Autodesk Inventor part; units mm, degrees
ref_plane "YZ Plane" through (0, 0, 0) normal (1, 0, 0) x (0, 1, 0)
ref_plane "XZ Plane" through (0, 0, 0) normal (0, 1, 0) x (-1, 0, 0)
ref_plane "XY Plane" through (0, 0, 0) normal (0, 0, 1) x (1, 0, 0)
sketch "Sketch1" plane through (0, 0, 0) normal (0, 0, 1) x (1, 0, 0)
  line L0 (-35.56, 38.35) -> (-35.56, 5)
  line L1 (0, 5) -> (0, 38.35)
  line L2 (-37.78, 47.225) -> (2.22, 47.225)
  line L3 (2.22, -2.775) -> (-37.78, -2.775)
  line L4 (-37.78, -2.775) -> (-37.78, 47.225)
  line L5 (1.22, 24.725) -> (1.22, 19.725)
  line L6 (1.22, 19.725) -> (2.22, 19.725)
  line L7 (2.22, 24.725) -> (1.22, 24.725)
  line L8 (2.22, 47.225) -> (2.22, 24.725)
  line L9 (2.22, 19.725) -> (2.22, -2.775)
  circle A0 centre (-3.05, 41.4) radius 1.4
  circle A1 centre (-32.51, 41.4) radius 1.4
  arc A2 (-6.1, 41.4) -> (-3.05, 38.35) centre (-3.05, 41.4) ccw
  line L10 (-6.1, 41.4) -> (-6.1, 44.45)
  line L11 (-3.05, 38.35) -> (0, 38.35)
  arc A3 (-32.51, 38.35) -> (-29.46, 41.4) centre (-32.51, 41.4) ccw
  line L12 (-29.46, 41.4) -> (-29.46, 44.45)
  line L13 (-32.51, 38.35) -> (-35.56, 38.35)
  line L14 (-6.1, 44.45) -> (-29.46, 44.45)
  line L15 (-35.56, 5) -> (0, 5)
  line L16 (0, 38.35) -> (0, 44.45)
  line L17 (0, 44.45) -> (-6.1, 44.45)
  line L18 (-29.46, 44.45) -> (-35.56, 44.45)
  line L19 (-35.56, 44.45) -> (-35.56, 38.35)
  line L20 (0, 5) -> (-35.56, 5)
  line L21 (-35.56, 5) -> (-35.56, -0.1476)
  line L22 (-35.56, -0.1476) -> (0, -0.1476)
  line L23 (0, -0.1476) -> (0, 5)
  point P0 (-17.78, 22.225)
  dimension "d0" = 40
  dimension "d1" = 50
  dimension "d2" = 5
  dimension "d4" = 1
  dimension "d6" = 7.775
  dimension "d8" = 3.05
  dimension "d9" = 2.8
extrude "Extrusion1" add sketch "Sketch1" along normal blind 5 contours L2 L8 L7 L5 L6 L9 L3 L4
ref_plane "Work Plane1" through (0, 0, 0) normal (0, 0, 1) x (1, 0, 0)
sketch "Sketch2" plane through (0, 0, 0) normal (0, 0, 1) x (1, 0, 0)
  line L0 (-35.56, 38.35) -> (-35.56, 5)
  line L1 (0, 5) -> (0, 38.35)
  line L2 (-37.78, 47.225) -> (2.22, 47.225)
  line L3 (2.22, -2.775) -> (-37.78, -2.775)
  line L4 (-37.78, -2.775) -> (-37.78, 47.225)
  line L5 (1.22, 24.725) -> (1.22, 19.725)
  line L6 (1.22, 19.725) -> (2.22, 19.725)
  line L7 (2.22, 24.725) -> (1.22, 24.725)
  line L8 (2.22, 47.225) -> (2.22, 24.725)
  line L9 (2.22, 19.725) -> (2.22, -2.775)
  circle A0 centre (-3.05, 41.4) radius 1.4
  circle A1 centre (-32.51, 41.4) radius 1.4
  arc A2 (-6.1, 41.4) -> (-3.05, 38.35) centre (-3.05, 41.4) ccw
  line L10 (-6.1, 41.4) -> (-6.1, 44.45)
  line L11 (-3.05, 38.35) -> (0, 38.35)
  arc A3 (-32.51, 38.35) -> (-29.46, 41.4) centre (-32.51, 41.4) ccw
  line L12 (-29.46, 41.4) -> (-29.46, 44.45)
  line L13 (-32.51, 38.35) -> (-35.56, 38.35)
  line L14 (-6.1, 44.45) -> (-29.46, 44.45)
  line L15 (-35.56, 5) -> (0, 5)
  line L16 (0, 38.35) -> (0, 44.45)
  line L17 (0, 44.45) -> (-6.1, 44.45)
  line L18 (-29.46, 44.45) -> (-35.56, 44.45)
  line L19 (-35.56, 44.45) -> (-35.56, 38.35)
  line L20 (0, 5) -> (-35.56, 5)
  line L21 (-35.56, 5) -> (-35.56, -0.2)
  line L22 (-35.56, -0.2) -> (0, -0.2)
  line L23 (0, -0.2) -> (0, 5)
  line L24 (-35.56, -0.1476) -> (0, -0.1476)
  point P0 (0, 0)
  point P1 (-17.78, 22.225)
  dimension "d12" = 40
  dimension "d13" = 50
  dimension "d14" = 5
  dimension "d15" = 1
  dimension "d16" = 7.775
  dimension "d17" = 3.05
  dimension "d18" = 2.8
  dimension "d27" = 5.2
extrude "Extrusion2" add sketch "Sketch2" along normal blind 2 contours L19 L18 L12 A3 L13 | L15 L23 L24 L21 | L24 L23 L22 L21 | L11 A2 L10 L17 L16
sketch "Sketch3" plane through (-37.78, -2.775, 0) normal (-1, 0, 0) x (0, 0, 1)
  line L0 (5.9421, 36.5891) -> (1.9421, 36.5891)
  line L1 (1.9421, 36.5891) -> (1.9421, 23.5891)
  line L2 (1.9421, 23.5891) -> (5.9421, 23.5891)
  line L3 (5.9421, 23.5891) -> (5.9421, 36.5891)
  point P0 (0, 2.775)
  dimension "d21" = 4
  dimension "d22" = 13
extrude "Extrusion3" cut sketch "Sketch3" against normal up to surface (2.22 mm away)
sketch "Sketch4" plane through (0, 0, 0) normal (0, 0, -1) x (-1, 0, 0)
  line L0 (9.525, 39.121) -> (2.794, 39.121)
  line L1 (2.794, 39.121) -> (2.0566, 39.0072)
  line L2 (2.0566, 39.0072) -> (1.3738, 38.7064)
  arc A0 (29.46, 41.4) -> (32.51, 38.35) centre (32.51, 41.4) ccw
  line L3 (30.483, 39.121) -> (32.766, 39.121)
  line L4 (35.56, 38.35) -> (32.51, 38.35)
  arc A1 (34.63, 38.35) -> (32.766, 39.121) centre (32.5832, 36.0404) ccw
  line L5 (34.63, 38.35) -> (32.51, 38.35)
  arc A2 (30.483, 39.121) -> (32.51, 38.35) centre (32.51, 41.4) ccw
  arc A3 (3.05, 38.35) -> (6.1, 41.4) centre (3.05, 41.4) ccw
  arc A4 (3.05, 38.35) -> (5.1075, 39.121) centre (3.078, 41.4062) ccw
  arc A5 (2.794, 39.121) -> (0.93, 38.35) centre (2.917, 36.1849) ccw
  line L6 (5.1075, 39.121) -> (2.794, 39.121)
  line L7 (3.05, 38.35) -> (0.93, 38.35)
  point P0 (0, 0)
extrude "Extrusion4" cut sketch "Sketch4" against normal blind 2 contours A4 A3 L0 | A3 L7 A5 L2 L1 L0 | L1 A5 | A5 L2 | L3 A1 L4 A0
sketch "Sketch5" plane through (0, 0, 0) normal (0, 0, -1) x (-1, 0, 0)
  line L0 (26.712, -2.7097) -> (26.628, -2.7097)
  line L1 (0, 5) -> (35.56, 5)
  line L2 (4.162, 5) -> (10.062, 5)
  line L3 (31.67, -2.775) -> (31.67, 5)
  line L4 (31.67, 5) -> (21.67, 5)
  line L5 (21.67, 5) -> (21.67, -2.775)
  line L6 (11.112, -2.775) -> (11.112, 5)
  line L7 (11.112, 5) -> (3.112, 5)
  line L8 (3.112, 5) -> (3.112, -2.775)
  line L9 (31.67, -2.775) -> (21.67, -2.775)
  line L10 (-2.22, -2.775) -> (37.78, -2.775)
  line L11 (11.112, -2.775) -> (3.112, -2.775)
  point P0 (0, 0)
  point P1 (26.67, -2.775)
  point P2 (7.112, -2.775)
extrude "Extrusion5" cut sketch "Sketch5" against normal blind 3.5 contours L1 L6 L10 L8 | L5 L1 L3 L9
sketch "Sketch6" plane through (0, 0, 0) normal (0, 0, -1) x (-1, 0, 0)
  line L0 (45.4266, 18.5636) -> (67.4266, 18.5636)
  line L1 (45.4266, -1.4364) -> (45.4266, 18.5636)
  line L2 (21.67, 3.8524) -> (21.67, -0.1476)
  line L3 (11.112, 3.8524) -> (11.112, -2.775)
  line L4 (11.112, -2.775) -> (21.67, -2.775)
  line L5 (21.67, -2.775) -> (21.67, 3.8524)
  line L6 (21.67, 3.8524) -> (11.112, 3.8524)
  line L7 (21.67, -2.775) -> (21.67, 5)
  point P0 (0, 0)
  dimension "d37" = 22
  dimension "d38" = 20
extrude "Extrusion6" add sketch "Sketch6" along normal blind 2 from surface at 0
For this review, take the finished solid that the model builds, in its own axes (mm). A direction names the side the tool comes from. Give positions to 0.01 mm unless a question says otherwise; leave off trailing zeros. Write each loop counter-clockwise with the first axis right and the second up, starting at its lowest first coordinate (ties: lowest second). Pieces come first, ordered by that corner, then holes. Notation, with made-up numbers: M -9.5,-39 L 5.5,-39 A13 ccw 5.5,-21 Z; hole C 33,9.5 d9. An arc over 180 degrees is marked long. One line per item, written item: value.
1) Take a section at A-A, the plane x = -25.5. Write out the cut boundary in (y, z) (3 decimals).
Results are:
outline: M -2.775,3.5 L -0.148,3.5 L -0.148,5 L -2.775,5 Z; M 44.45,0 L 47.225,0 L 47.225,5 L 44.45,5 Z
2) Take a section at C-C, the plane y = 2. Write out the cut boundary in (x, z).
Results are:
outline: M -37.78,0 L -31.67,0 L -31.67,2 L -35.56,2 L -35.56,5 L -37.78,5 Z; M -21.67,-2 L -11.11,-2 L -11.11,2 L -21.67,2 Z; M -3.11,0 L 2.22,0 L 2.22,5 L 0,5 L 0,2 L -3.11,2 Z
3) For P1, Ø2, axis at x = -29.5, y = 41.5, coming from the +Z side; P2, Ø1.3, axis at x = -25, y = -2, coming from the -Z side; P3, Ø1, axis at x = -4, z = 1, coming from the -Y side; P4, Ø6, axis at x = -6, y = 36, coming from the -Z side, all flat-tipped, find the tip position at first contact; note any pin that passes through.
Results are:
P1: stops at z = 2
P2: stops at z = 3.5
P3: stops at y = 39.12
P4: passes through
4) For faces 5 (the flat face through (2, 19.725, 2)), 6 (the flat face through (-3.112, 0, 1)), 7 (the flat face through (-16, 5, 1)), 8 (the cylindrical face through (-29.72, 40.17, 0.99)), 9 (the flat face through (-33, 43, 2)), list the 3-axis set-ups (+Z, -Z, +X, -X, +Y, -Y) from which the entire face can be reached by the end or side of a thin tool; tool diameter is ignored.
Results are:
face 5: +Z, -Z, +X
face 6: -Z, -Y
face 7: +Z, -Z
face 8: +Z, -Z, -Y
face 9: +Z
5) The part is to be moulded in two halves that separate along Y. For faces 1 (the flat face through (-16, 3.852, -1)), 2 (the flat face through (-18, -2.775, 2)), 3 (the flat face through (2, 24.725, 2)), 4 (the flat face through (-7, -1, 3.5)), say which applies: +Y half, -Y half, draft (parallel to the pull), parting line (faces both ways), or undercut.
Results are:
face 1: +Y half
face 2: -Y half
face 3: undercut
face 4: draft
6) For line 1 (Y direction, x = -3.05, z = 0.85) (3 decimals); line 2 (Y direction, x = -9.5, z = 4.5) (3 decimals); line 3 (Y direction, x = -14.5, z = 0.75) (3 decimals), list the stretches that pass through material, from the lowest coordinate up. Write a range as from..to.
Results are:
line 1: y = -2.775..5, 39.121..40, 42.8..47.225
line 2: y = -2.775..-0.148, 44.45..47.225
line 3: y = -2.775..5, 44.45..47.225
7) Take a section at B-B, the plane y = 32. Write out the cut boundary in (x, z).
Results are:
outline: M -37.78,0 L -35.56,0 L -35.56,1.94 L -37.78,1.94 Z; M 0,0 L 2.22,0 L 2.22,5 L 0,5 Z
